Geometry: see drawing. Coordinates: mm, zero at the bounding-box minimum. A direction names the side the tool comes from. Give positions to 0.01 mm unless a question says otherwise; leave off trailing zeros. Order: outer loops, then holes, each group sorted by start corner. A loop starts at its lowest first (then second) coordinate and runs counter-clockwise, first axis right, second up. Notation, with made-up numbers: M -19.75,-23 L 38.25,-23 A17 ccw 38.25,4 Z; hole C 35,64.25 d8. An arc over 180 degrees is marked long. Use a Markdown table: item, result.
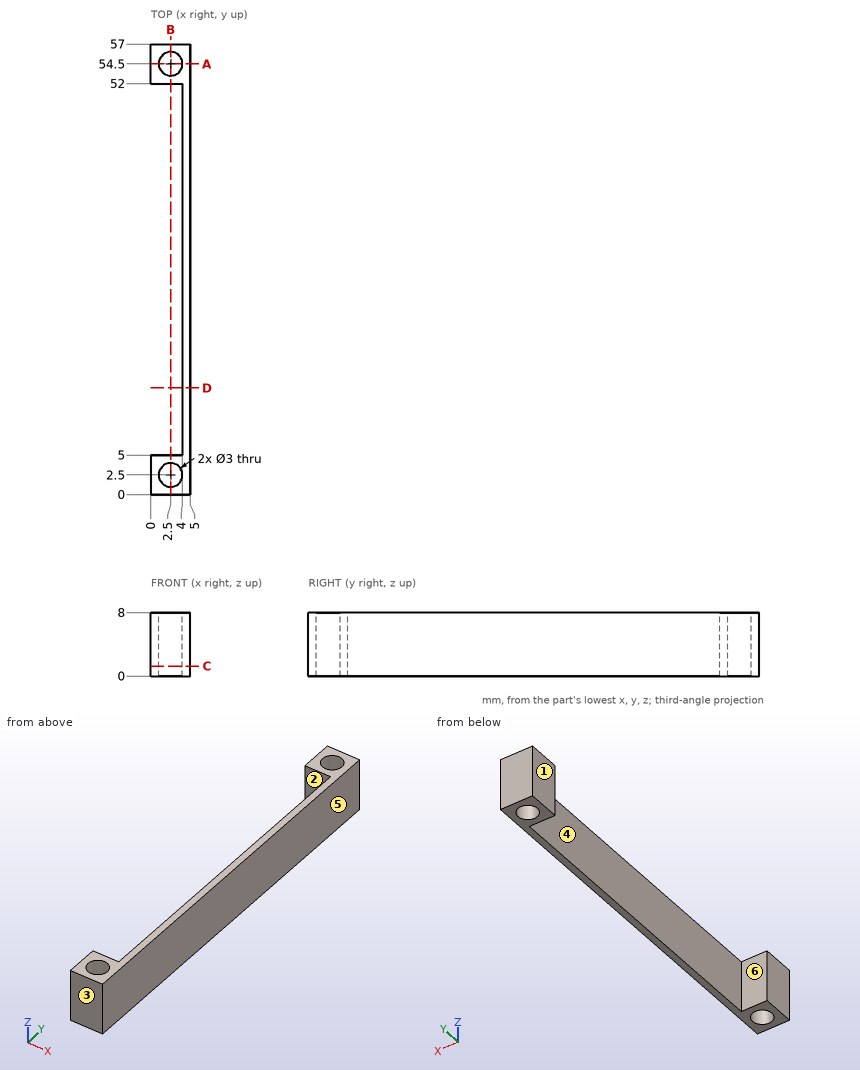
1) Material intervals for line 1 (Y direction, x = 2.5, z = 4.5); line 2 (Y direction, x = 3.75, z = 7.75); line 3 (X direction, y = 31, z = 7), sorted ascending. Write a range as from..to.
Response values:
| item | result |
|---|---|
| line 1 | y = 0..1, 4..5, 52..53, 56..57 |
| line 2 | y = 0..1.67, 3.33..5, 52..53.67, 55.33..57 |
| line 3 | x = 4..5 |
2) Cut plane B-B on x = 2.5. Return loops of the section in (y, z).
Response values:
| item | result |
|---|---|
| outline | M 0,0 L 1,0 L 1,8 L 0,8 Z; M 4,0 L 5,0 L 5,8 L 4,8 Z; M 52,0 L 53,0 L 53,8 L 52,8 Z; M 56,0 L 57,0 L 57,8 L 56,8 Z |
3) Mould query, pull axis Y, two halves, no side actions, for the marked faces 1, 2, 3 and 4. Classes: released by +Y, released by -Y, zero draft, split by the parting line, or undercut.
Response values:
| item | result |
|---|---|
| face 1 | zero draft |
| face 2 | undercut |
| face 3 | released by -Y |
| face 4 | undercut |
4) Cut plane D-D on y = 13.5. Return loops of the section in (x, z).
Response values:
| item | result |
|---|---|
| outline | M 4,0 L 5,0 L 5,8 L 4,8 Z |
5) First-contact query: pin 1 Ø4 at (y, z) = (18, 4.5) entering from -X. Flat tip, straight axial feed; report the tip coordinate or a pass-through.
Response values:
| item | result |
|---|---|
| pin 1 | stops at x = 4 |
6) Cut plane C-C on z = 1.25. Return loops of the section in (x, y), and give its area (3 significant figures).
Response values:
| item | result |
|---|---|
| outline | M 0,0 L 5,0 L 5,57 L 0,57 L 0,52 L 4,52 L 4,5 L 0,5 Z; hole C 2.5,2.5 d3; hole C 2.5,54.5 d3 |
| area | 82.9 mm² |
7) Cut plane A-A on y = 54.5. Return loops of the section in (x, z).
Response values:
| item | result |
|---|---|
| outline | M 0,0 L 1,0 L 1,8 L 0,8 Z; M 4,0 L 5,0 L 5,8 L 4,8 Z |
8) Reachability of the marked faces 5 and 6 from +Z, -Z, +X, -X, +Y, -Y: full face, straight path, thin tool, end or side. Return the list, or none.
Response values:
| item | result |
|---|---|
| face 5 | +Z, -Z, +X, +Y, -Y |
| face 6 | +Z, -Z, -X |
